from build123d import *

# Parameters (mm, degrees)
SKETCH1_R           = 7.5
BOSS_EXTRUDE1_DEPTH = 6
BOSS_EXTRUDE2_START = -3
SKETCH2_R           = 10
SKETCH2_R_2         = 7.5
BOSS_EXTRUDE2_DEPTH = 3
FILLET1_R           = 3
SKETCH3_R           = 3
CUT_EXTRUDE1_DEPTH  = 16.362291496


with BuildPart() as part:
    # Sketch1 → Boss-Extrude1 (new body)
    with BuildSketch(Plane(origin=(0, 0, 0), x_dir=(1, 0, 0), z_dir=(0, 1, 0))):
        with Locations(Location((0, 0, 0), (0, 0, 270))):
            Circle(SKETCH1_R)
    extrude(amount=BOSS_EXTRUDE1_DEPTH)

    # Sketch2 → Boss-Extrude2 (add)
    with BuildSketch(Plane(origin=(0, 6, 0), x_dir=(1, 0, 0), z_dir=(0, 1, 0)).offset(BOSS_EXTRUDE2_START)):
        with Locations(Location((0, 0, 0), (0, 0, 270))):
            Circle(SKETCH2_R)
        with Locations(Location((0, 0, 0), (0, 0, 270))):
            Circle(SKETCH2_R_2, mode=Mode.SUBTRACT)
    extrude(amount=BOSS_EXTRUDE2_DEPTH)

    # Fillet1
    fillet1_edges = [part.edges().sort_by_distance(p)[0] for p in [
        (0, 6, -10),
    ]]
    fillet(fillet1_edges, radius=FILLET1_R - 0.0001)  # a hair under: the kernel refuses the full size

    # Sketch3 → Cut-Extrude1 (cut, through all)
    with BuildSketch(Plane(origin=(0, 6, 0), x_dir=(1, 0, 0), z_dir=(0, 1, 0))):
        with Locations(Location((0, 0, 0), (0, 0, 270))):
            Circle(SKETCH3_R)
    extrude(amount=-CUT_EXTRUDE1_DEPTH, mode=Mode.SUBTRACT)


solid = part.part
Work out the finished part from the listing and answer in its coordinate system (mm). Round coordinates to 2 decimals unless told otherwise and drop trailing zeros. Loops run counter-clockwise (first coordinate to the right, second up) from the corner with the lowest first, then second, coordinate; pieces in that order, holes last. Notation, with made-up numbers: (42, 80.5) -> (76, 80.5) arc R21 cw to (76, 113.5) -> close; hole circle Ø4 at (36.25, 74). An arc over 180 degrees is marked (long way). Use one line per item in the form item = value.
(1) Find section C-C on y = 1.7. Give the vertices of the cut face in (x, z), then the cut area to 3 significant figures.
Answer list:
outline = circle Ø15 at (0, 0); hole circle Ø6 at (0, 0)
area = 148 mm2
(2) Flat-ended cylindrical pins translate along their axes: P1, Ø1.5, axis at y = 4, z = 6, coming from the +X side; P2, Ø2, axis at x = -0.5, y = 1.5, coming from the +Z side; P3, Ø4, axis at x = 3, z = 6, coming from the -Y side. Find the tip coordinate at first contact, or state that the pin passes through.
Answer list:
P1 = 8.37
P2 = 7.5
P3 = 0
(3) Straight lines are drawn through the part: line 1 (X direction, y = 2.5, z = 0); line 2 (X direction, y = 3.15, z = 0.25); line 3 (Z direction, x = -2.5, y = 3.05). For each, find the intervals that lie inside material, in ascending order.
Answer list:
line_1 = -7.5 to -3, 3 to 7.5
line_2 = -9.99 to -2.99, 2.99 to 9.99
line_3 = -9.68 to -1.66, 1.66 to 9.68
(4) Find section D-D on y = 5.05. Give the vertices of the cut face in (x, z).
Answer list:
outline = circle Ø18.38 at (0, 0); hole circle Ø6 at (0, 0)
(5) For a pull along Z with two mould halves and no side action, classify faces 1 (the flat face through (7, 3, 4)), 2 (the cylindrical face through (0.9, 3.04, 2.86)), 3 (the cylindrical face through (0.33, 1.479, -7.493)) as released by +Z, released by -Z, zero draft, split by the parting line, or undercut.
Answer list:
face_1 = zero draft
face_2 = undercut
face_3 = split by the parting line
